```python
from build123d import *

# Parameters (mm, degrees)
F0_R         = 2.3495
F1_DEPTH     = 15.6718
F3_R         = 2.5273
F4_DEPTH     = 0.5588
F5_DEPTH     = 12.7
F6_R         = 2.9464
F7_DEPTH     = 8.5598
F8_R         = 12.7
F9_DEPTH     = 7.9502
F10_W        = 1.4605
F10_H        = 1.8034
F10_W_2      = 1.8034
F10_H_2      = 1.4605
F11_DEPTH    = 7.2898
F12_T1_DEPTH = 7.9030102448
F13_R        = 0.6745312693
F14_R        = 1.7145
F15_DEPTH    = 5.8674


# Not quite as in the source:
# - a fillet or chamfer that OpenCascade refuses, or shapes differently, is made with other operations: its cross-section is extruded or revolved along the edge and cut away or added


with BuildPart() as f1:
    # F0 (on Top) → F1 (new body)
    with BuildSketch(Plane.XY):
        Circle(F0_R)
    extrude(amount=F1_DEPTH)

    # F3 (on face) → F4 (join)
    with BuildSketch(Plane(origin=(0, 0, 0), x_dir=(1, 0, 0), z_dir=(0, 0, -1))):
        Circle(F3_R)
    extrude(amount=-F4_DEPTH)

    # F2 (on Front) → F5 (cut, symmetric)
    with BuildSketch(Plane.XZ):
        with BuildLine():
            Line((-0.5461, -2.8702), (0.5461, -2.8702))
            Line((0.5461, -2.8702), (0.5461, 2.8702))
            ThreePointArc((0.5461, 2.8702), (0, 2.3241), (-0.5461, 2.8702))
            Line((-0.5461, 2.8702), (-0.5461, -2.8702))
        make_face()
        with BuildLine():
            ThreePointArc((-0.5461, 2.8702), (0, 2.3241), (0.5461, 2.8702))
            Line((0.5461, 2.8702), (-0.5461, 2.8702))
        make_face()
        with BuildLine():
            Line((-0.5461, 2.8702), (0.5461, 2.8702))
            ThreePointArc((0.5461, 2.8702), (0, 3.4163), (-0.5461, 2.8702))
        make_face()
    extrude(amount=F5_DEPTH, both=True, mode=Mode.SUBTRACT)

    # F6 (on face) → F7 (join)
    with BuildSketch(Plane.XY.offset(15.6718)):
        Circle(F6_R)
    extrude(amount=-F7_DEPTH)

    # F8 (on face) → F9 (cut)
    with BuildSketch(Plane.XY.offset(15.6718)):
        Circle(F8_R)
    extrude(amount=-F9_DEPTH, mode=Mode.SUBTRACT)

    # F10 (on face) → F11 (join)
    with BuildSketch(Plane.XY.offset(7.7216)):
        with Locations((1.63195, 0)):
            Rectangle(F10_W, F10_H)
        with Locations((0, -1.63195)):
            Rectangle(F10_W_2, F10_H_2)
        Rectangle(F10_W_2, F10_H)
        with Locations((-1.63195, 0)):
            Rectangle(F10_W, F10_H)
        with Locations((0, 1.63195)):
            Rectangle(F10_W_2, F10_H_2)
    extrude(amount=F11_DEPTH)

    # F12: fillet of radius 0.2452840979 on 4 edges, made by hand

    # F12_s2 → F12_t1 (join)
    with BuildSketch(Plane.XY.offset(7.1083897552)):
        with BuildLine():
            add(Edge.make_bspline(
                [(-1.1469840979, -0.9017), (-0.9017, -0.9017), (-0.9017, -1.1469840979)],
                knots=[0, 0, 0, 1, 1, 1], degree=2, weights=[1, 1, 1]))
            Line((-0.9017, -1.1469840979), (-0.9017, -0.9017))
            Line((-0.9017, -0.9017), (-1.1469840979, -0.9017))
        make_face()
        with BuildLine():
            add(Edge.make_bspline(
                [(1.1469840979, 0.9017), (0.9017, 0.9017), (0.9017, 1.1469840979)],
                knots=[0, 0, 0, 1, 1, 1], degree=2, weights=[1, 1, 1]))
            Line((0.9017, 1.1469840979), (0.9017, 0.9017))
            Line((0.9017, 0.9017), (1.1469840979, 0.9017))
        make_face()
        with BuildLine():
            add(Edge.make_bspline(
                [(1.1469840979, -0.9017), (0.9017, -0.9017), (0.9017, -1.1469840979)],
                knots=[0, 0, 0, 1, 1, 1], degree=2, weights=[1, 1, 1]))
            Line((0.9017, -1.1469840979), (0.9017, -0.9017))
            Line((0.9017, -0.9017), (1.1469840979, -0.9017))
        make_face()
        with BuildLine():
            add(Edge.make_bspline(
                [(-0.9017, 1.1469840979), (-0.9017, 0.9017), (-1.1469840979, 0.9017)],
                knots=[0, 0, 0, 1, 1, 1], degree=2, weights=[1, 1, 1]))
            Line((-1.1469840979, 0.9017), (-0.9017, 0.9017))
            Line((-0.9017, 0.9017), (-0.9017, 1.1469840979))
        make_face()
    extrude(amount=F12_T1_DEPTH)

    # F13
    f13_edges = [f1.edges().sort_by_distance(p)[0] for p in [
        (1.754592, -0.9017, 15.0114),
        (2.3622, 0, 15.0114),
        (1.754592, 0.9017, 15.0114),
        (0.963022, 0.96302, 15.0114),
        (0.9017, 1.754592, 15.0114),
        (0, 2.3622, 15.0114),
        (-0.9017, 1.754592, 15.0114),
        (-0.96302, 0.963022, 15.0114),
        (-1.754592, 0.9017, 15.0114),
        (-2.3622, 0, 15.0114),
        (-1.754592, -0.9017, 15.0114),
        (-0.963022, -0.96302, 15.0114),
        (-0.9017, -1.754592, 15.0114),
        (0, -2.3622, 15.0114),
        (0.9017, -1.754592, 15.0114),
        (0.963022, -0.96302, 15.0114),
    ]]
    fillet(f13_edges, radius=F13_R)

    # F14 (on face) → F15 (cut)
    with BuildSketch(Plane(origin=(0, 0, 0), x_dir=(1, 0, 0), z_dir=(0, 0, -1))):
        Circle(F14_R)
    extrude(amount=-F15_DEPTH, mode=Mode.SUBTRACT)


solid = f1.part
```
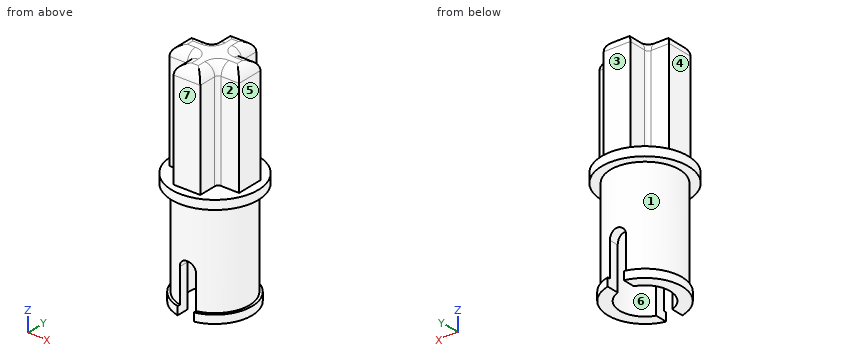
Design review of the part built by this model. Coordinates are the model's own, in mm. Face numbers are marked on the shaded views. A direction names the side the tool comes from. Give positions to 0.01 mm unless a question says otherwise; leave off trailing zeros. Order: outer loops, then holes, each group sorted by start corner. A loop starts at its lowest first (then second) coordinate and runs counter-clockwise, first axis right, second up. Notation, with made-up numbers: (-13.5, 63) - (3.5, 63) arc R15 cw to (3.5, 78) - close; hole circle Ø10 at (50, -36.75). An arc over 180 degrees is marked (long way). Use a Markdown table: item, result. Add a question column.
(1) Add section A-A on y = 0. Give the boundary of the cut face in (x, z).
(2) Clearance check with flat-ended pins moving along their axes: P1, Ø2, axis at x = -2, y = 1, coming from the -Z side; P2, Ø1.3, axis at y = -1.5, z = 12, coming from the -X side; P3, Ø1.4, axis at y = 0, z = 11, coming from the +X side; P4, Ø1, axis at x = 2, z = 10, coming from the +Y side. State where each tip first meets the part, or that it passes through.
(3) Add section C-C on x = 0. Give the boundary of the cut face in (y, z).
(4) Mouldability with a two-part tool opening along Y and no side actions: class the marked faces 5, 6 and 7 as +Y half, -Y half, draft (parallel to the pull), parting line (faces both ways), or undercut.
(5) Wall thickness on probe 1 along Y at (x, z) = (0, 4.65); probe 2 along Y at (x, z) = (1.25, 8): over which ranges is each line inside the solid? List them lowest first. Write a range as [from, to].
(6) Add section D-D on z = 4.75. Give the boundary of the cut face in (x, y), then the cut area to 3 significant figures.
(7) Add section B-B on z = 2.25. Give the boundary of the cut face in (x, y), then the cut area to 3 significant figures.
(8) Machinability: for the marked faces 1, 2, 3 and 4, which of the approach directions +Z, -Z, +X, -X, +Y, -Y give a long, thin tool a straight path to every point of the face, cutting with its end or side? Answer none if there is none.
Report:
| question | item | result |
|---|---|---|
| 1 | outline | (-2.95, 7.11) - (-2.35, 7.11) - (-2.35, 0.56) - (-2.53, 0.56) - (-2.53, 0) - (-1.71, 0) - (-1.71, 5.87) - (1.71, 5.87) - (1.71, 0) - (2.53, 0) - (2.53, 0.56) - (2.35, 0.56) - (2.35, 7.11) - (2.95, 7.11) - (2.95, 7.72) - (2.36, 7.72) - (2.36, 14.34) arc R0.67 ccw to (1.69, 15.01) - (-1.69, 15.01) arc R0.67 ccw to (-2.36, 14.34) - (-2.36, 7.72) - (-2.95, 7.72) - close |
| 2 | P1 | stops at z = 0 |
| 2 | P2 | stops at x = -2.36 |
| 2 | P3 | stops at x = 2.36 |
| 2 | P4 | stops at y = 0.9 |
| 3 | outline | (-2.95, 7.11) - (-2.35, 7.11) - (-2.35, 3.42) - (-1.71, 3.42) - (-1.71, 5.87) - (1.71, 5.87) - (1.71, 3.42) - (2.35, 3.42) - (2.35, 7.11) - (2.95, 7.11) - (2.95, 7.72) - (2.36, 7.72) - (2.36, 14.34) arc R0.67 ccw to (1.69, 15.01) - (-1.69, 15.01) arc R0.67 ccw to (-2.36, 14.34) - (-2.36, 7.72) - (-2.95, 7.72) - close |
| 4 | face 5 | draft |
| 4 | face 6 | undercut |
| 4 | face 7 | -Y half |
| 5 | probe 1 | y = [-2.35, -1.71], [1.71, 2.35] |
| 5 | probe 2 | y = [-0.9, 0.9] |
| 6 | outline | circle Ø4.7 at (0, 0); hole circle Ø3.43 at (0, 0) |
| 6 | area | 8.11 mm² |
| 7 | outline | (-0.55, -2.29) - (-0.55, -1.63) arc R1.71 cw to (-0.55, 1.63) - (-0.55, 2.29) arc R2.35 ccw to start; (0.55, -2.29) arc R2.35 ccw to (0.55, 2.29) - (0.55, 1.63) arc R1.71 cw to (0.55, -1.63) - close |
| 7 | area | 6.70 mm² |
| 8 | face 1 | none |
| 8 | face 2 | +Z, +X, -Y |
| 8 | face 3 | +Z, +X, -X, +Y |
| 8 | face 4 | +Z, -X, +Y, -Y |
